Study the drawing (mm; zero at the part's minimum x, y, z) and answer. A direction names the side the tool comes from. Coordinates: 2 decimals unless noted, no trailing zeros. Order: outer loops, then holes, each group sorted by start corner. A loop starts at its lowest first (then second) coordinate and runs counter-clockwise, first axis right, second up. Notation, with made-up numbers: M -5,79.25 L 52,79.25 A9 cw 52,86.25 Z; hole C -16,-4 d11. An arc over 180 degrees is marked long. Use a Markdown table: item, result. Add a question column.
1) Find section A-A on x = 12.7. Write down the section's boundary in (y, z) (1 decimal), plus the area to 3 significant figures.
2) For the marked faces 1 and 2, determine the directions among +Z, -Z, +X, -X, +Y, -Y from which every point of the face is accessible in a straight line to the end or side of a thin tool.
3) The mould has two halves that part along X. Classify the marked faces 3, 4, 5 and 6: released by +X, released by -X, zero draft, split by the parting line, or undercut.
4) Find section C-C on x = 20.32. Write down the section's boundary in (y, z) (1 decimal).
5) Find section B-B on y = 2. Write down the section's boundary in (x, z).
6) Find section D-D on z = 3.9. Count the separate pieces of the cut face and the enclosed holes in it.
7) This flat-tipped pin is pushed along its axis until it touches: pin 1 Ø1 at (x, y) = (16, 26.5) entering from -Z. Where does it stop, or does it pass through?
8) Find the intervals of material crossed by probe 1 along Y at (x, z) = (12.7, 1.1) (1 decimal); probe 2 along X at (y, z) = (4.5, 4.4); probe 3 along Y at (x, z) = (5.08, 3.3) (1 decimal), in increasing order. Write a range as [from, to].
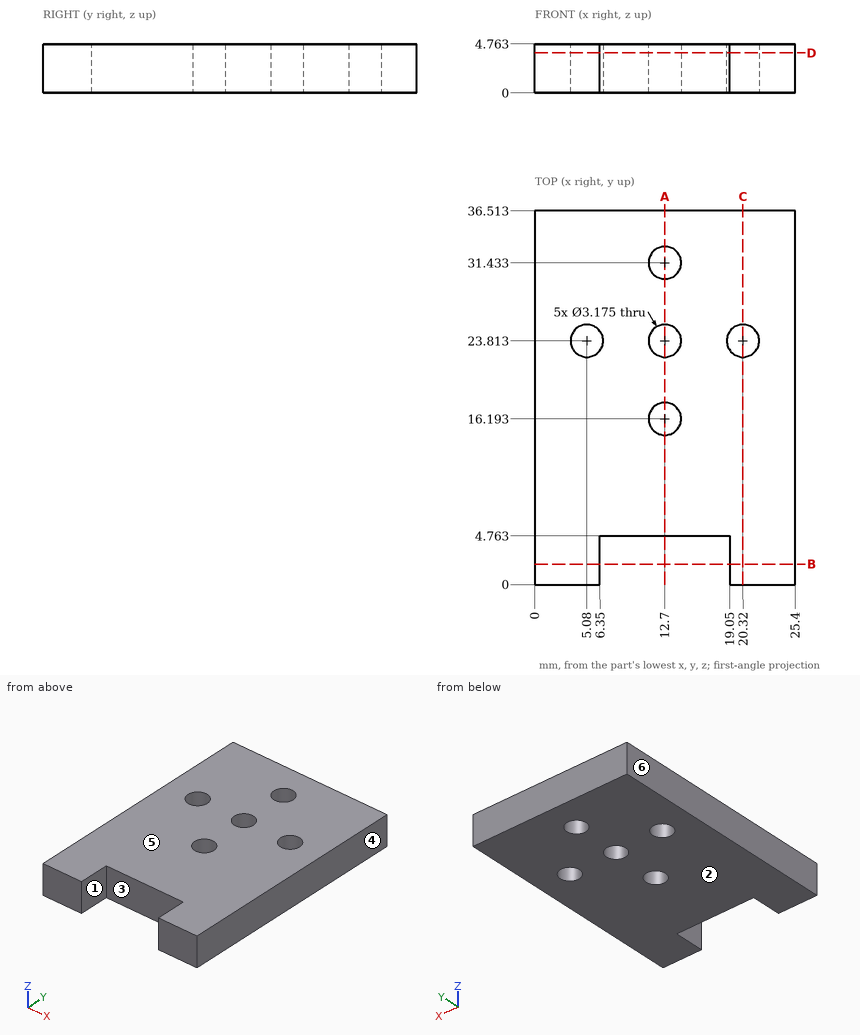
Check result:
| question | item | result |
|---|---|---|
| 1 | outline | M 4.8,0 L 14.6,0 L 14.6,4.8 L 4.8,4.8 Z; M 17.8,0 L 22.2,0 L 22.2,4.8 L 17.8,4.8 Z; M 25.4,0 L 29.8,0 L 29.8,4.8 L 25.4,4.8 Z; M 33,0 L 36.5,0 L 36.5,4.8 L 33,4.8 Z |
| 1 | area | 106 mm2 |
| 2 | face 1 | +Z, -Z, -Y |
| 2 | face 2 | -Z, +X, -X, +Y, -Y |
| 3 | face 3 | undercut |
| 3 | face 4 | released by +X |
| 3 | face 5 | zero draft |
| 3 | face 6 | released by -X |
| 4 | outline | M 0,0 L 22.2,0 L 22.2,4.8 L 0,4.8 Z; M 25.4,0 L 36.5,0 L 36.5,4.8 L 25.4,4.8 Z |
| 5 | outline | M 0,0 L 6.35,0 L 6.35,4.76 L 0,4.76 Z; M 19.05,0 L 25.4,0 L 25.4,4.76 L 19.05,4.76 Z |
| 6 | separate pieces | 1 |
| 6 | enclosed holes | 5 |
| 7 | pin 1 | stops at z = 0 |
| 8 | probe 1 | y = [4.8, 14.6], [17.8, 22.2], [25.4, 29.8], [33, 36.5] |
| 8 | probe 2 | x = [0, 6.35], [19.05, 25.4] |
| 8 | probe 3 | y = [0, 22.2], [25.4, 36.5] |
